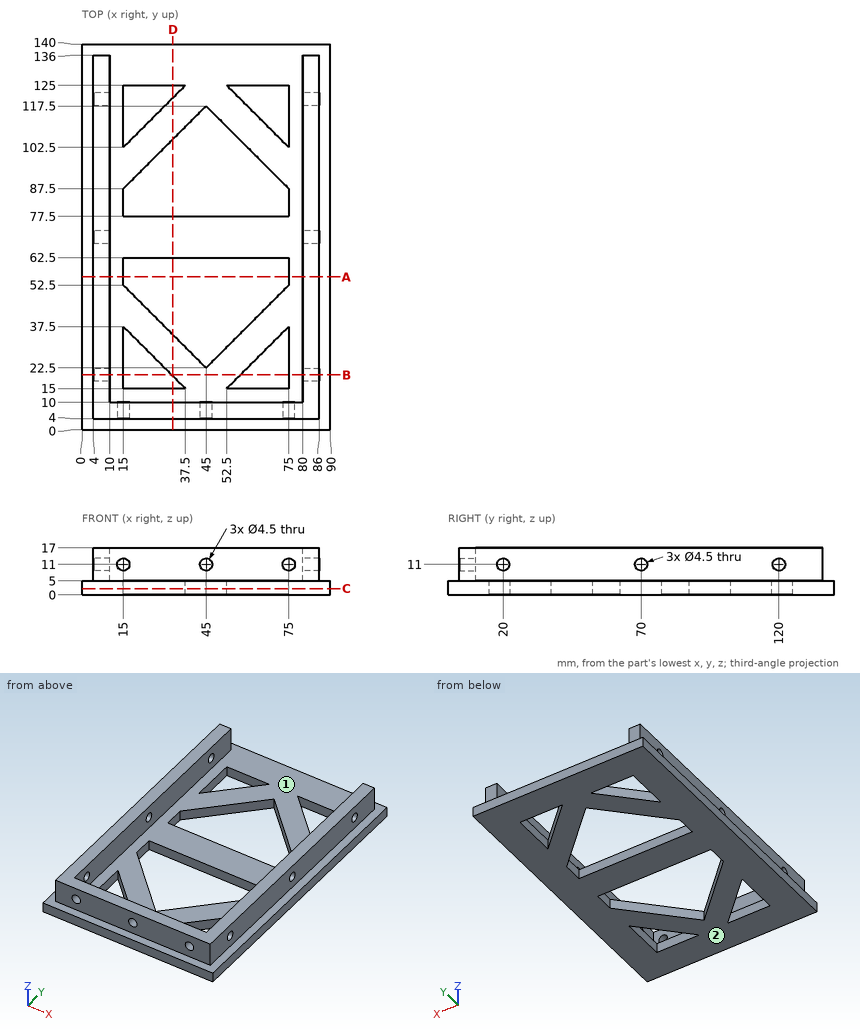
Job drawing, mm, ordinate dimensions from the low corner. One solid piece. Coordinates: 2 decimals unless noted, no trailing zeros. Write each loop counter-clockwise with the first axis right and the second up, starting at its lowest first coordinate (ties: lowest second). Pieces come first, ordered by that corner, then holes. Notation, with made-up numbers: (22.5, 32.5) - (64.5, 32.5) arc R15 ccw to (64.5, 52.5) - close; hole circle Ø9 at (-4, -39). An arc over 180 degrees is marked (long way). Use a Markdown table: item, result. Add a question column.
Item 1: Flat gauge pins, fed straight in: pin 1 (6 mm diameter, centred on x = 75, y = 41.5, fed in from +Z); pin 2 (3.5 mm diameter, centred on y = 120, z = 11, fed in from +X); pin 3 (5.5 mm diameter, centred on x = 46, z = 3, fed in from -Y); pin 4 (3.5 mm diameter, centred on x = 52, z = 10.5, fed in from -Y). Where does each tip first touch, or does it go through?
Item 2: Band-saw the part on C-C, the plane z = 2.25. Give the cut face in (x, y).
Item 3: Band-saw the part on D-D, the plane x = 33. Give the cut face in (y, z).
Item 4: Band-saw the part on A-A, the plane y = 55.5. Give the cut face in (x, z).
Item 5: Band-saw the part on B-B, the plane y = 20. Give the cut face in (x, z).
Item 6: Mould opens along X. For the marked faces 1 and 2 say: pulls with the +X half, pulls with the -X half, needs draft (parallel to the pull), parting line crosses it, or undercut.
Item 7: Drill centre lines: L1, parallel to X at y = 114, z = 7.75; L2, parallel to Z at x = 5.7, y = 120; L3, parallel to Y at x = 56.5, z = 2.5. Where is each one in solid material? Low to high. Write a range as from..to.
Numbers:
| question | item | result |
|---|---|---|
| 1 | pin 1 | z = 5 |
| 1 | pin 2 | through |
| 1 | pin 3 | y = 0 |
| 1 | pin 4 | y = 4 |
| 2 | outline | (0, 0) - (90, 0) - (90, 140) - (0, 140) - close; hole (15, 15) - (37.5, 15) - (15, 37.5) - close; hole (15, 52.5) - (45, 22.5) - (75, 52.5) - (75, 62.5) - (15, 62.5) - close; hole (15, 77.5) - (75, 77.5) - (75, 87.5) - (45, 117.5) - (15, 87.5) - close; hole (15, 102.5) - (37.5, 125) - (15, 125) - close; hole (52.5, 15) - (75, 15) - (75, 37.5) - close; hole (52.5, 125) - (75, 102.5) - (75, 125) - close |
| 3 | outline | (0, 0) - (15, 0) - (15, 5) - (10, 5) - (10, 17) - (4, 17) - (4, 5) - (0, 5) - close; (19.5, 0) - (34.5, 0) - (34.5, 5) - (19.5, 5) - close; (62.5, 0) - (77.5, 0) - (77.5, 5) - (62.5, 5) - close; (105.5, 0) - (120.5, 0) - (120.5, 5) - (105.5, 5) - close; (125, 0) - (140, 0) - (140, 5) - (125, 5) - close |
| 4 | outline | (0, 0) - (15, 0) - (15, 5) - (10, 5) - (10, 17) - (4, 17) - (4, 5) - (0, 5) - close; (75, 0) - (90, 0) - (90, 5) - (86, 5) - (86, 17) - (80, 17) - (80, 5) - (75, 5) - close |
| 5 | outline | (0, 0) - (15, 0) - (15, 5) - (10, 5) - (10, 8.75) - (4, 8.75) - (4, 5) - (0, 5) - close; (4, 13.25) - (10, 13.25) - (10, 17) - (4, 17) - close; (32.5, 0) - (57.5, 0) - (57.5, 5) - (32.5, 5) - close; (75, 0) - (90, 0) - (90, 5) - (86, 5) - (86, 8.75) - (80, 8.75) - (80, 5) - (75, 5) - close; (80, 13.25) - (86, 13.25) - (86, 17) - (80, 17) - close |
| 6 | face 1 | undercut |
| 6 | face 2 | needs draft |
| 7 | L1 | 4..10, 80..86 |
| 7 | L2 | 0..8.75, 13.25..17 |
| 7 | L3 | 0..15, 19..34, 62.5..77.5, 106..121, 125..140 |
